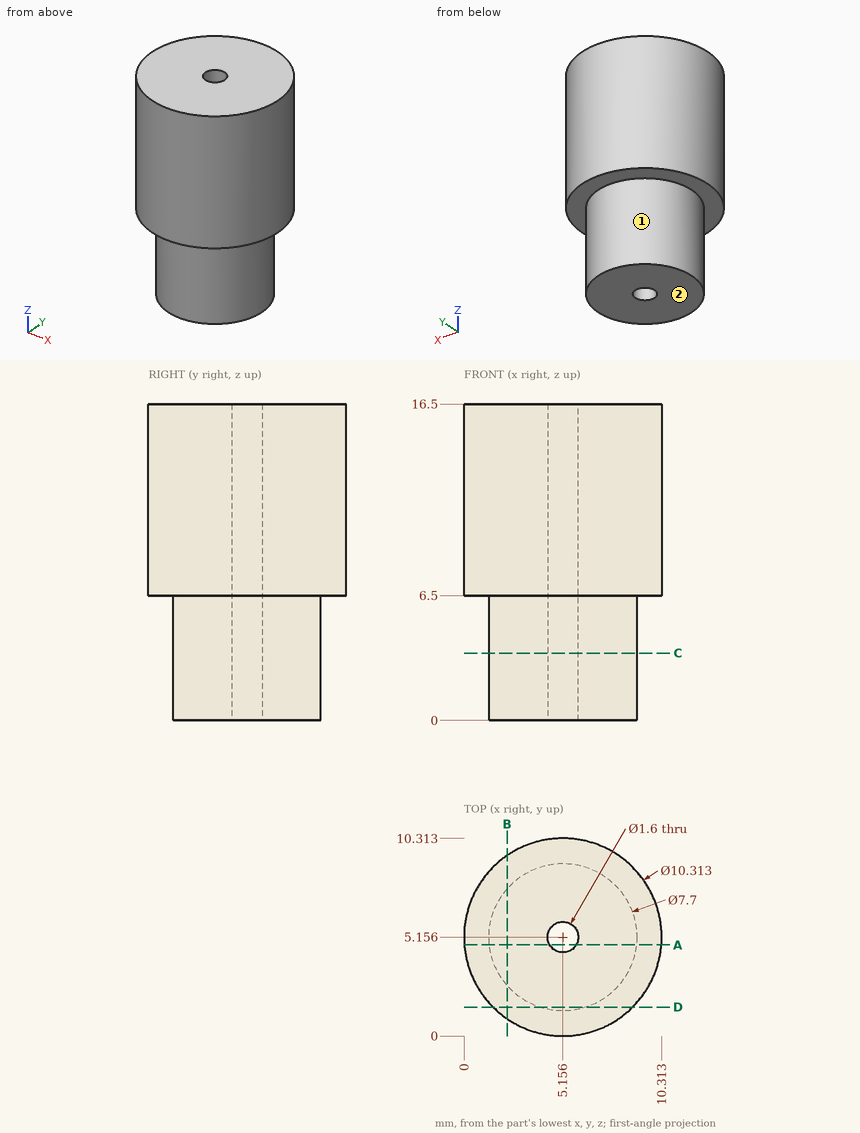
For this review, use the dimensioned drawing (mm, ordinates from the lowest corner) and the shaded views. A direction names the side the tool comes from. Give positions to 0.01 mm unless a question says otherwise; leave off trailing zeros. Order: outer loops, then holes, each group sorted by start corner. A loop starts at its lowest first (then second) coordinate and runs counter-clockwise, first axis right, second up. Notation, with made-up numbers: (9, -26.75) - (33, -26.75) arc R18 ccw to (33, -6.75) - close; hole circle Ø6 at (71, 80.5). An arc over 180 degrees is marked (long way). Use a Markdown table: item, result. Add a question column.
(1) Clearance check with flat-ended pins moving along their axes: P1, Ø1.3, axis at x = 5.16, y = 5.16, coming from the -Z side; P2, Ø1, axis at y = 7.5, z = 12, coming from the +X side. State where each tip first meets the part, or that it passes through.
(2) Add section A-A on y = 4.75. Give the boundary of the cut face in (x, z) (1 decimal).
(3) Add section B-B on x = 2.25. Give the boundary of the cut face in (y, z) (1 decimal), then the cut area to 3 significant figures.
(4) Add section D-D on y = 1.5. Give the boundary of the cut face in (x, z).
(5) Wall thickness on probe 1 along Y at (x, z) = (5.5, 11.75) (1 decimal); probe 2 along X at (y, z) = (4.75, 3.75) (1 decimal); probe 3 along Z at (x, y) = (9, 2): over which ranges is each line inside the solid? List them lowest first. Write a range as [from, to].
(6) Add section C-C on z = 3.5. Give the boundary of the cut face in (x, y).
(7) Machinability: for the marked faces 1 and 2, which of the approach directions +Z, -Z, +X, -X, +Y, -Y give a long, thin tool a straight path to every point of the face, cutting with its end or side? Answer none if there is none.
Report:
| question | item | result |
|---|---|---|
| 1 | P1 | passes through |
| 1 | P2 | stops at x = 9.97 |
| 2 | outline | (0, 6.5) - (1.3, 6.5) - (1.3, 0) - (4.5, 0) - (4.5, 16.5) - (0, 16.5) - close; (5.8, 0) - (9, 0) - (9, 6.5) - (10.3, 6.5) - (10.3, 16.5) - (5.8, 16.5) - close |
| 3 | outline | (0.9, 6.5) - (2.6, 6.5) - (2.6, 0) - (7.7, 0) - (7.7, 6.5) - (9.4, 6.5) - (9.4, 16.5) - (0.9, 16.5) - close |
| 3 | area | 118 mm² |
| 4 | outline | (1.52, 6.5) - (3.95, 6.5) - (3.95, 0) - (6.36, 0) - (6.36, 6.5) - (8.79, 6.5) - (8.79, 16.5) - (1.52, 16.5) - close |
| 5 | probe 1 | y = [0, 4.4], [5.9, 10.3] |
| 5 | probe 2 | x = [1.3, 4.5], [5.8, 9] |
| 5 | probe 3 | z = [6.5, 16.5] |
| 6 | outline | circle Ø7.7 at (5.16, 5.16); hole circle Ø1.6 at (5.16, 5.16) |
| 7 | face 1 | -Z |
| 7 | face 2 | -Z, +X, -X, +Y, -Y |
